from build123d import *

# Parameters (mm, degrees)
SKETCH1_R           = 19
BOSS_EXTRUDE1_DEPTH = 10
SKETCH2_R           = 2.5
CUT_EXTRUDE1_DEPTH  = 10
CUT_EXTRUDE2_DEPTH  = 10


with BuildPart() as part:
    # Sketch1 → Boss-Extrude1 (new body)
    with BuildSketch(Plane.XY):
        Circle(SKETCH1_R)
    extrude(amount=BOSS_EXTRUDE1_DEPTH)

    # Sketch2 → Cut-Extrude1 (cut)
    with BuildSketch(Plane.XY.offset(10)):
        Circle(SKETCH2_R)
    extrude(amount=-CUT_EXTRUDE1_DEPTH, mode=Mode.SUBTRACT)

    # Sketch3 → Cut-Extrude2 (cut)
    with BuildSketch(Plane.XY.offset(10)):
        with BuildLine():
            ThreePointArc((-3.299671038, 3.059766501), (-2.25, 3.897114317), (-1, 4.387482194))
            Line((-1, 4.387482194), (-1, 16.970562748))
            ThreePointArc((-1, 16.970562748), (-8.5, 14.722431864), (-14.196938457, 9.351306778))
            Line((-14.196938457, 9.351306778), (-3.299671038, 3.059766501))
        make_face()
        with BuildLine():
            ThreePointArc((-4.299671038, -1.327715693), (-4.5, 0), (-4.299671038, 1.327715693))
            Line((-4.299671038, 1.327715693), (-15.196938457, 7.61925597))
            ThreePointArc((-15.196938457, 7.61925597), (-17, 0), (-15.196938457, -7.61925597))
            Line((-15.196938457, -7.61925597), (-4.299671038, -1.327715693))
        make_face()
        with BuildLine():
            ThreePointArc((-1, -4.387482194), (-2.25, -3.897114317), (-3.299671038, -3.059766501))
            Line((-3.299671038, -3.059766501), (-14.196938457, -9.351306778))
            ThreePointArc((-14.196938457, -9.351306778), (-8.5, -14.722431864), (-1, -16.970562748))
            Line((-1, -16.970562748), (-1, -4.387482194))
        make_face()
        with BuildLine():
            Line((14.196938457, -9.351306778), (3.299671038, -3.059766501))
            ThreePointArc((3.299671038, -3.059766501), (2.25, -3.897114317), (1, -4.387482194))
            Line((1, -4.387482194), (1, -16.970562748))
            ThreePointArc((1, -16.970562748), (8.5, -14.722431864), (14.196938457, -9.351306778))
        make_face()
        with BuildLine():
            Line((15.196938457, 7.61925597), (4.299671038, 1.327715693))
            ThreePointArc((4.299671038, 1.327715693), (4.449635922, 0.671371852), (4.5, 0))
            ThreePointArc((4.5, 0), (4.449635922, -0.671371852), (4.299671038, -1.327715693))
            Line((4.299671038, -1.327715693), (15.196938457, -7.61925597))
            ThreePointArc((15.196938457, -7.61925597), (16.543094538, -3.9148465), (17, 0))
            ThreePointArc((17, 0), (16.543094538, 3.9148465), (15.196938457, 7.61925597))
        make_face()
        with BuildLine():
            Line((1, 16.970562748), (1, 4.387482194))
            ThreePointArc((1, 4.387482194), (2.25, 3.897114317), (3.299671038, 3.059766501))
            Line((3.299671038, 3.059766501), (14.196938457, 9.351306778))
            ThreePointArc((14.196938457, 9.351306778), (8.5, 14.722431864), (1, 16.970562748))
        make_face()
    extrude(amount=-CUT_EXTRUDE2_DEPTH, mode=Mode.SUBTRACT)


solid = part.part
Check sheet for the modelled part. Datum: model origin and axes. Units: mm. A direction names the side the tool comes from. Round coordinates to 2 decimals unless told otherwise and drop trailing zeros. Loops run counter-clockwise (first coordinate to the right, second up) from the corner with the lowest first, then second, coordinate; pieces in that order, holes last.
1. Sectioned sample at C-C on y = 13. Record the boundary of the cut face in (x, z), and give its area (3 significant figures).
2. Sectioned sample at A-A on z = 5.75. Record the boundary of the cut face in (x, y).
3. Sectioned sample at D-D on x = 11. Record the boundary of the cut face in (y, z), and give its area (3 significant figures).
4. Sectioned sample at B-B on x = 0. Record the boundary of the cut face in (y, z).
5. Set-up check for faces 1 (the cylindrical face through (8, -15, 5)), 2 (the flat face through (0, -4, 0)): record each of +Z, -Z, +X, -X, +Y, -Y from which the full face is reachable in a straight line by a thin tool's end or side.
6. Scan lines: probe 1 along Y at (x, z) = (0, 7.75); probe 2 along X at (y, z) = (-10.5, 8.25); probe 3 along X at (y, z) = (10, 4). Record each from-to range of solid material in increasing order.
7. Gauge pin test, flat ends, axial feed: pin 1 Ø4.5 at (x, y) = (0, 0) entering from -Z; pin 2 Ø3 at (y, z) = (2, 7.5) entering from +X; pin 3 Ø3 at (y, z) = (-11.5, 4.5) entering from +X; pin 4 Ø6 at (x, z) = (7.5, 8) entering from -Y. Record the tip position at first contact, or that the pin passes through.
8. Mould release check, pull along Y, two halves, no side actions. Record for faces 3 (the flat face through (-1, -11, 5)), 4 (the flat face through (0, -4, 10)): released by +Y, released by -Y, zero draft, split by the parting line, or undercut.
Recorded:
1. outline: (-13.86, 0) - (-10.95, 0) - (-10.95, 10) - (-13.86, 10) - close; (-1, 0) - (1, 0) - (1, 10) - (-1, 10) - close; (10.95, 0) - (13.86, 0) - (13.86, 10) - (10.95, 10) - close
1. area: 78.0 mm2
2. outline: circle Ø38 at (0, 0); hole (-15.2, -7.62) - (-4.3, -1.33) arc R4.5 cw to (-4.3, 1.33) - (-15.2, 7.62) arc R17 ccw to start; hole (-14.2, -9.35) arc R17 ccw to (-1, -16.97) - (-1, -4.39) arc R4.5 cw to (-3.3, -3.06) - close; hole (-14.2, 9.35) - (-3.3, 3.06) arc R4.5 cw to (-1, 4.39) - (-1, 16.97) arc R17 ccw to start; hole circle Ø5 at (0, 0); hole (1, -16.97) arc R17 ccw to (14.2, -9.35) - (3.3, -3.06) arc R4.5 cw to (1, -4.39) - close; hole (1, 4.39) arc R4.5 cw to (3.3, 3.06) - (14.2, 9.35) arc R17 ccw to (1, 16.97) - close; hole (4.3, -1.33) - (15.2, -7.62) arc R17 ccw to (15.2, 7.62) - (4.3, 1.33) arc R4.5 cw to start
3. outline: (-15.49, 0) - (-12.96, 0) - (-12.96, 10) - (-15.49, 10) - close; (-7.51, 0) - (-5.2, 0) - (-5.2, 10) - (-7.51, 10) - close; (5.2, 0) - (7.51, 0) - (7.51, 10) - (5.2, 10) - close; (12.96, 0) - (15.49, 0) - (15.49, 10) - (12.96, 10) - close
3. area: 96.8 mm2
4. outline: (-19, 0) - (-2.5, 0) - (-2.5, 10) - (-19, 10) - close; (2.5, 0) - (19, 0) - (19, 10) - (2.5, 10) - close
5. face 1: +Z, -Z
5. face 2: -Z, +X, -X, +Y, -Y
6. probe 1: y = -19 to -2.5, 2.5 to 19
6. probe 2: x = -15.84 to -13.37, -1 to 1, 13.37 to 15.84
6. probe 3: x = -16.16 to -13.75, -1 to 1, 13.75 to 16.16
7. pin 1: passes through
7. pin 2: stops at x = 18.99
7. pin 3: stops at x = 16.16
7. pin 4: stops at y = -18.46
8. face 3: undercut
8. face 4: zero draft
